Build history of the part. All positions in model axes, mm. A direction names the side the tool comes from. Round coordinates to 2 decimals unless told otherwise and drop trailing zeros. Order: outer loops, then holes, each group sorted by start corner. A loop starts at its lowest first (then second) coordinate and runs counter-clockwise, first axis right, second up. Notation, with made-up numbers: (-12, -1) -> (27, -1) arc R8 cw to (27, 14) -> close; hole circle Ø10 at (72, 5). An arc over 180 degrees is marked (long way). Write item = value, one per line.
from build123d import *

# Parameters (mm, degrees)
M3_GEWINDEBOHRUNG1_D     = 2.5
M3_GEWINDEBOHRUNG1_DEPTH = 6.5
M3_GEWINDEBOHRUNG1_TIP   = 0.751075774
FASE1_SIZE               = 0.2
SKETCH2_R                = 1.25
CUT_EXTRUDE1_DEPTH       = 3


# Read off the part's stored shape, not the designer's step: M2.5 Machine Threads Stud1
with BuildPart() as part:
    # Skizze1 → Rotation1 (revolve)
    with BuildSketch(Plane.XY, mode=Mode.PRIVATE) as rotation1_sk:
        Polygon((19, 0), (-16, 0), (-16, 2), (16, 2), (16, 1.25), (19, 1.25), align=None)
    revolve(rotation1_sk.sketch.rotate(Axis((0, 0, 0), (1, 0, 0)), 90), axis=Axis((0, 0, 0), (1, 0, 0)))

    # M3 Gewindebohrung1
    with Locations(Plane.ZY.offset(16)):
        with Locations((0, 0)):
            Hole(M3_GEWINDEBOHRUNG1_D / 2, depth=M3_GEWINDEBOHRUNG1_DEPTH)
            with Locations((0, 0, -(M3_GEWINDEBOHRUNG1_DEPTH + M3_GEWINDEBOHRUNG1_TIP / 2))):  # 118° drill point
                Cone(0, M3_GEWINDEBOHRUNG1_D / 2, M3_GEWINDEBOHRUNG1_TIP, mode=Mode.SUBTRACT)

    # Fase1
    fase1_edges = [part.edges().sort_by_distance(p)[0] for p in [
        (19, 0, -1.25),
    ]]
    chamfer(fase1_edges, length=FASE1_SIZE)

    # Sketch2 → Cut-Extrude1 (cut)
    with BuildSketch(Plane(origin=(19, 0, 0), x_dir=(0, 0, -1), z_dir=(1, 0, 0))):
        with Locations(Location((0, 0, 0), (0, 0, 180))):
            Circle(SKETCH2_R)
    extrude(amount=-CUT_EXTRUDE1_DEPTH, mode=Mode.SUBTRACT)

    # M2.5 Machine Threads Stud1 outline → M2.5 Machine Threads Stud1 (revolve)
    with BuildSketch(Plane.YX):
        Polygon((0.9965, 21), (0, 21), (0, 16), (1.25, 16), (1.25, 20.7465), align=None)
    revolve(axis=Axis((0, 0, 0), (1, 0, 0)))


solid = part.part
Q1. Cut at B-B, the plane x = 12.5. List the corners of the cut face in (y, z), and give its area (3 significant figures).
Check values:
outline = circle Ø4 at (0, 0)
area = 12.6 mm²
Q2. Cut at A-A, the plane y = 1.6. List the corners of the cut face in (x, z), and give its area (3 significant figures).
Check values:
outline = (-16, -1.2) -> (16, -1.2) -> (16, 1.2) -> (-16, 1.2) -> close
area = 76.8 mm²
Q3. Probe probe 1 along Y at (x, z) = (-14.25, 0); probe 2 along X at (y, z) = (0.05, 1.55); probe 3 along Y at (x, z) = (-8, 0.1). List the from-to ranges inside material, lowest first.
Check values:
probe_1 = -2 to -1.25, 1.25 to 2
probe_2 = -16 to 16
probe_3 = -2 to 2
Q4. Flat gauge pins, fed straight in: pin 1 (1.5 mm diameter, centred on x = 16, z = 1.5, fed in from -Y); pin 2 (1.5 mm diameter, centred on x = -3.5, z = -1, fed in from -Y); pin 3 (1 mm diameter, centred on x = 8.5, z = 0.5, fed in from +Y). Where does each tip first touch, or does it go through?
Check values:
pin_1 = -1.85
pin_2 = -1.98
pin_3 = 2
Q5. Mould opens along Z. For faces 1 (the face through (0, 2, 0)), 2 (the face through (16, -1, 1)), 3 (the face through (-8.88, -0.21, -0.05)), 4 (the face through (-12.7, -1.22, 0.27)) say: released by +Z, released by -Z, zero draft, split by the parting line, or undercut.
Check values:
face_1 = split by the parting line
face_2 = zero draft
face_3 = undercut
face_4 = undercut
Q6. Which spindle directions (+Z, -Z, +X, -X, +Y, -Y) get a long thin tool onto all of the face, cutting with end or side? Do faces 5 (the face through (-16, -1, -1)), 6 (the face through (18.41, -0.27, -1.22)). Say none if no direction does.
Check values:
face_5 = +Z, -Z, -X, +Y, -Y
face_6 = +X
